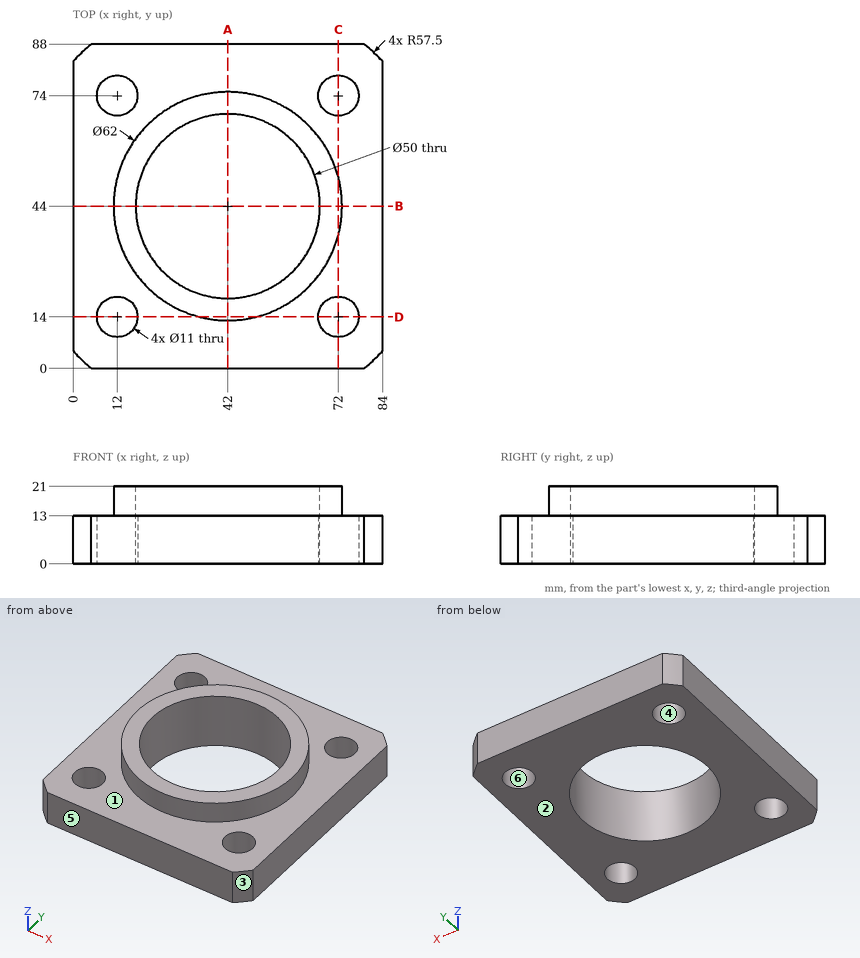
Check sheet for the drawn part. Datum: minimum x, y, z corner. Units: mm. A direction names the side the tool comes from. Give positions to 0.01 mm unless a question says otherwise; leave off trailing zeros. Order: outer loops, then holes, each group sorted by start corner. A loop starts at its lowest first (then second) coordinate and runs counter-clockwise, first axis right, second up. Notation, with made-up numbers: (55.5, 14.5) - (99.5, 14.5) arc R29 cw to (99.5, 45.5) - close; hole circle Ø1 at (33, -33). An arc over 180 degrees is marked (long way). Answer in a Markdown table with one row per item. Add a question column.
Q1. Tool access check on the marked faces 1 and 2. Record the directions out of +Z, -Z, +X, -X, +Y, -Y that give a thin tool (end or side, any length) a straight path to the whole face; none if there is none.
Q2. Gauge pin test, flat ends, axial feed: pin 1 (5 mm diameter, centred on x = 30.5, z = 16, fed in from -Y) (1 decimal); pin 2 (14.5 mm diameter, centred on x = 12, y = 74, fed in from +Z); pin 3 (2 mm diameter, centred on x = 41.5, z = 14.5, fed in from -Y). Record the tip position at first contact, or that the pin passes through.
Q3. Cross-section at C-C, the plane x = 72. Enter the section's corners in (y, z).
Q4. Cross-section at A-A, the plane x = 42. Enter the section's corners in (y, z).
Q5. Mould release check, pull along X, two halves, no side actions. Record for the marked faces 3, 4, 5 and 6: pulls with the +X half, pulls with the -X half, needs draft (parallel to the pull), parting line crosses it, or undercut.
Q6. Cross-section at D-D, the plane y = 14. Enter the section's corners in (x, z).
Q7. Material ranges on probe 1 along Y at (x, z) = (72, 6.75); probe 2 along Y at (x, z) = (13.5, 2.75); probe 3 along Y at (x, z) = (42, 11.5), recorded low to high. Write a range as from..to.
Q8. Cross-section at B-B, the plane y = 44. Enter the section's corners in (x, z).
Check values:
| question | item | result |
|---|---|---|
| 1 | face 1 | +Z |
| 1 | face 2 | -Z, +X, -X, +Y, -Y |
| 2 | pin 1 | stops at y = 14.3 |
| 2 | pin 2 | stops at z = 13 |
| 2 | pin 3 | stops at y = 13 |
| 3 | outline | (0, 0) - (8.5, 0) - (8.5, 13) - (0, 13) - close; (19.5, 0) - (68.5, 0) - (68.5, 13) - (51.81, 13) - (51.81, 21) - (36.19, 21) - (36.19, 13) - (19.5, 13) - close; (79.5, 0) - (88, 0) - (88, 13) - (79.5, 13) - close |
| 4 | outline | (0, 0) - (19, 0) - (19, 21) - (13, 21) - (13, 13) - (0, 13) - close; (69, 0) - (88, 0) - (88, 13) - (75, 13) - (75, 21) - (69, 21) - close |
| 5 | face 3 | pulls with the +X half |
| 5 | face 4 | undercut |
| 5 | face 5 | needs draft |
| 5 | face 6 | undercut |
| 6 | outline | (0, 0) - (6.5, 0) - (6.5, 13) - (0, 13) - close; (17.5, 0) - (66.5, 0) - (66.5, 13) - (49.81, 13) - (49.81, 21) - (34.19, 21) - (34.19, 13) - (17.5, 13) - close; (77.5, 0) - (84, 0) - (84, 13) - (77.5, 13) - close |
| 7 | probe 1 | y = 0..8.5, 19.5..68.5, 79.5..88 |
| 7 | probe 2 | y = 0..8.71, 19.29..68.71, 79.29..88 |
| 7 | probe 3 | y = 0..19, 69..88 |
| 8 | outline | (0, 0) - (17, 0) - (17, 21) - (11, 21) - (11, 13) - (0, 13) - close; (67, 0) - (84, 0) - (84, 13) - (73, 13) - (73, 21) - (67, 21) - close |
